Here's how the part is built. I have some questions about the finished solid (model axes, mm). Round coordinates to 2 decimals unless told otherwise and drop trailing zeros. Order: outer loops, then holes, each group sorted by start corner. A loop starts at its lowest first (then second) coordinate and runs counter-clockwise, first axis right, second up. Notation, with made-up numbers: M 50.5,66 L 79.5,66 A18 cw 79.5,72 Z; hole C 71,28.25 d8. An arc over 180 degrees is marked long. Answer as CSV lines item,"result". Start each with the question number.
```python
from build123d import *

# Parameters (mm, degrees)
SKETCH045_W     = 80
SKETCH045_H     = 55
PAD012_DEPTH    = 2
SKETCH046_R     = 1.75
POCKET037_DEPTH = 5
CHAMFER_SIZE    = 1


with BuildPart() as part:
    # Sketch045 → Pad012 (new body)
    with BuildSketch(Plane.XZ):
        with Locations((0, 27.5)):
            Rectangle(SKETCH045_W, SKETCH045_H)
    extrude(amount=PAD012_DEPTH)

    # Sketch046 (on Face5 of Pad012) → Pocket037 (cut)
    with BuildSketch(Plane(origin=(0, 0, 0), x_dir=(1, 0, 0), z_dir=(0, 1, 0))):
        with Locations((-36, -3.5)):
            Circle(SKETCH046_R)
        with Locations((-30, -51)):
            Circle(SKETCH046_R)
    pocket037 = extrude(amount=-POCKET037_DEPTH, mode=Mode.SUBTRACT)

    # Mirrored001: Pocket037 across Sketch046 V_Axis
    add(pocket037.mirror(Plane.YZ), mode=Mode.SUBTRACT)

    # Chamfer
    chamfer_edges = [part.edges().sort_by_distance(p)[0] for p in [
        (40, 0, 27.5),
        (0, 0, 55),
        (0, 0, 0),
        (-40, 0, 27.5),
        (40, -1, 55),
        (-40, -1, 55),
        (-40, -1, 0),
        (40, -1, 0),
    ]]
    chamfer(chamfer_edges, length=CHAMFER_SIZE)


with BuildPart() as part_1:
    # Body004 placement: moved
    add(part.part.moved(Location((0, 42, 0))))


solid = part_1.part
```
Item 1: If we section it at B-B on y = 41.5: Please give me the cut outline in (x, z).
Item 2: We'd pull the mould along X, two halves only. Please class faces 1 (the cylindrical face through (-34.383, 41.014, 4.17)), 2 (the flat face through (-1, 42, 28)): pulls with the +X half, pulls with the -X half, needs draft (parallel to the pull), parting line crosses it, or undercut.
Item 3: If I drill on line 1 along X through (y, z) = (41, 51); line 2 along X through (y, z) = (40.55, 3.5); line 3 along Z through (x, y) = (36, 40.75), over which ranges is the centre line in solid material (lowest first)?
Item 4: If we section it at C-C on x = -30: Please give me the cut outline in (y, z), and give its area (3 significant figures).
Item 5: If we section it at A-A on z = 3.5: Please give me the cut outline in (x, y).
Geometry says:
1,outline,"M -39.5,1 L -39,0.5 L 39,0.5 L 39.5,1 L 39.5,54 L 39,54.5 L -39,54.5 L -39.5,54 Z; hole C -36,3.5 d3.5; hole C -30,51 d3.5; hole C 30,51 d3.5; hole C 36,3.5 d3.5"
2,face 1,"undercut"
2,face 2,"needs draft"
3,line 1,"-40 to -31.75, -28.25 to 28.25, 31.75 to 40"
3,line 2,"-40 to -37.75, -34.25 to 34.25, 37.75 to 40"
3,line 3,"0 to 1.75, 5.25 to 55"
4,outline,"M 40,0 L 41,0 L 42,1 L 42,49.25 L 40,49.25 Z; M 40,52.75 L 42,52.75 L 42,54 L 41,55 L 40,55 Z"
4,area,"102 mm²"
5,outline,"M -40,40 L -37.75,40 L -37.75,42 L -39,42 L -40,41 Z; M -34.25,40 L 34.25,40 L 34.25,42 L -34.25,42 Z; M 37.75,40 L 40,40 L 40,41 L 39,42 L 37.75,42 Z"
